Autodesk Inventor part; units mm, degrees
ref_plane "YZ Plane" through (0, 0, 0) normal (1, 0, 0) x (0, 1, 0)
ref_plane "XZ Plane" through (0, 0, 0) normal (0, 1, 0) x (-1, 0, 0)
ref_plane "XY Plane" through (0, 0, 0) normal (0, 0, 1) x (1, 0, 0)
sketch "スケッチ1" plane through (0, 0, 0) normal (0, 1, 0) x (-1, 0, 0)
  arc A0 (-0.3139, 1.7491) -> (-1.4341, -1.0494) centre (0, 0) ccw
  arc A1 (3.0473, 2.0538) -> (-0.3139, 1.7491) centre (3.11, -17.328) ccw
  arc A2 (14.2243, 1.5555) -> (3.0473, 2.0538) centre (3.426, -115.066) ccw
  arc A3 (14.2243, 1.5555) -> (21.0741, 0.9324) centre (210.779, 2124.35) ccw
  arc A4 (21.0741, 0.9324) -> (33.8498, 0.3962) centre (33.144, 136.034) ccw
  arc A5 (33.8498, 0.3962) -> (55, 2.3978) centre (33.229, 119.698) ccw
  arc A6 (-1.4341, -1.0494) -> (-0.1426, -2.3034) centre (2.9, 2.122) ccw
  arc A7 (-0.1426, -2.3034) -> (4.4066, -4.5379) centre (9.743, 12.075) ccw
  arc A8 (4.4066, -4.5379) -> (12.2873, -5.9387) centre (13.508, 23.796) ccw
  arc A9 (12.2873, -5.9387) -> (16.5781, -5.9878) centre (15.261, 66.497) ccw
  arc A10 (16.5781, -5.9878) -> (55, 2.3978) centre (14.7503, 94.6026) ccw
  dimension "d0" = 1.777
  dimension "d2" = 17.328
  dimension "d5" = 115.066
  dimension "d7" = 2124.35
  dimension "d9" = 136.034
  dimension "d10" = 3.11
  dimension "d11" = 3.426
  dimension "d12" = 210.779
  dimension "d13" = 33.144
  dimension "d14" = 33.229
  dimension "d15" = 119.698
  dimension "d16" = 55
  dimension "d17" = 2.9
  dimension "d18" = 2.122
  dimension "d21" = 9.743
  dimension "d22" = 12.075
  dimension "d23" = 13.508
  dimension "d24" = 23.796
  dimension "d25" = 15.261
  dimension "d26" = 66.497
  dimension "d27" = 94.6026
extrude "押し出し1" add sketch "スケッチ1" along normal mid plane 95
properties part number "naca97"
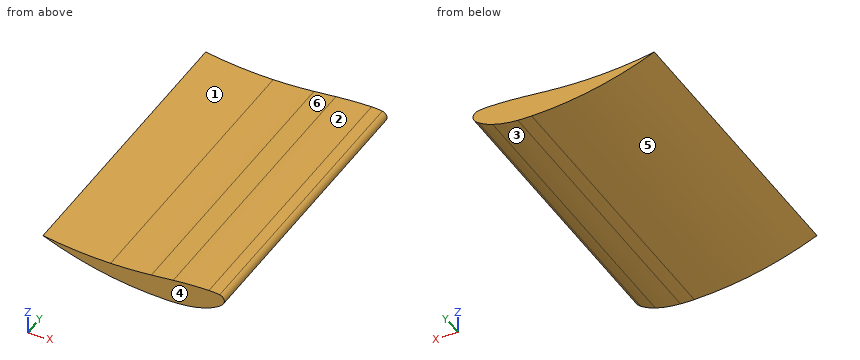
The listing builds one solid part. Answer for the finished solid, in the listing's coordinates (mm). Face numbers are marked on the shaded views. A direction names the side the tool comes from. Coordinates: 2 decimals unless noted, no trailing zeros. Write each loop counter-clockwise with the first axis right and the second up, starting at its lowest first coordinate (ties: lowest second). Pieces come first, ordered by that corner, then holes. Notation, with made-up numbers: M -22,-20.5 L -7,-20.5 A31 cw -7,17.5 Z; hole C 4.5,71 d5. An arc over 180 degrees is marked long. Put each result on its own line as item: value. Start each with the question number.
1. A cutting plane is placed at C-C on x = -29.5. Write down the section's boundary in (y, z).
2. A cutting plane is placed at B-B on x = -45.5. Write down the section's boundary in (y, z), then the cut area to 3 significant figures.
3. Consider line 1 (Z direction, x = -22.5, y = -1.5); line 2 (Z direction, x = -22, y = -34.5). Determine where each line is inside the solid, lowest interval first. Write a range as from..to.
4. Which of the six approach directions +Z, -Z, +X, -X, +Y, -Y give full straight-line access (tool end or side, diameter ignored) to the marked faces 5 and 6?
5. For a pull along X with two mould halves and no side action, classify the marked faces 1, 2, 3 and 4 as pulls with the +X half, pulls with the -X half, needs draft (parallel to the pull), parting line crosses it, or undercut.
6. Flat-ended cylindrical pins translate along their axes: P1, Ø1.5, axis at y = 36, z = -3.5, coming from the +X side; P2, Ø5, axis at x = -44, y = 15, coming from the -Z side; P3, Ø3, axis at x = -45.5, y = 3.5, coming from the +Z side. Find the tip coordinate at first contact, or state that the pin passes through.
7. A cutting plane is placed at A-A on y = -32. Write down the section's boundary in (x, z), then the cut area to 3 significant figures.
Resolved:
1. outline: M -47.5,-4.92 L 47.5,-4.92 L 47.5,0.44 L -47.5,0.44 Z
2. outline: M -47.5,-1.19 L 47.5,-1.19 L 47.5,1.03 L -47.5,1.03 Z
2. area: 211 mm2
3. line 1: z = -5.71..0.81
3. line 2: z = -5.74..0.85
4. face 5: -Z, -X, +Y, -Y
4. face 6: +Z, +Y, -Y
5. face 1: undercut
5. face 2: undercut
5. face 3: pulls with the +X half
5. face 4: needs draft
6. P1: stops at x = -0.54
6. P2: stops at z = -2.38
6. P3: stops at z = 1.19
7. outline: M -55,2.4 A100.61 ccw -16.58,-5.99 A72.56 ccw -12.29,-5.94 A29.76 ccw -4.41,-4.54 A17.45 ccw 0.14,-2.3 A5.37 ccw 1.43,-1.05 A1.78 ccw 0.31,1.75 A19.38 ccw -3.05,2.05 A117.15 ccw -14.22,1.56 A2133.11 cw -21.07,0.93 A135.62 cw -33.85,0.4 A119.31 cw Z
7. area: 275 mm2
